```python
from build123d import *

# Parameters (mm, degrees)
SKETCH1_R           = 1.5
BOSS_EXTRUDE1_DEPTH = 3
SKETCH3_R           = 8.6
CUT_EXTRUDE2_DEPTH  = 4
SKETCH4_R           = 1.5
SKETCH4_R_2         = 1.475
CUT_EXTRUDE3_DEPTH  = 4
CUT_EXTRUDE4_DEPTH  = 4
CUT_EXTRUDE6_DEPTH  = 4
CUT_EXTRUDE7_DEPTH  = 4


with BuildPart() as part:
    # Sketch1 → Boss-Extrude1 (new body)
    with BuildSketch(Plane.XY):
        Polygon((0, -20.476245627), (7.465897773, -20.476245627), (9.02146997, -21.374355653), (9.387495374, -22.740381057), (11.136866689, -23.750381057), (15.4496732, -26.240381057), (21.596787517, -24.59326674), (32.096787517, -6.40673326), (30.4496732, -0.259618943), (26.136866689, 2.230381057), (24.387495374, 3.240381057), (23.02146997, 2.874355653), (21.465897773, 3.772465679), (17.732948887, 10.238122813), (14, 16.703779947), (14, 18.5), (15, 19.5), (15, 23), (15, 26.5), (10.5, 31), (-10.5, 31), (-15, 26.5), (-15, 23), (-15, 19.5), (-14, 18.5), (-14, 16.703779947), (-17.732948887, 10.238122813), (-21.465897773, 3.772465679), (-23.02146997, 2.874355653), (-24.387495374, 3.240381057), (-26.136866689, 2.230381057), (-30.4496732, -0.259618943), (-32.096787517, -6.40673326), (-21.596787517, -24.59326674), (-15.4496732, -26.240381057), (-11.136866689, -23.750381057), (-9.387495374, -22.740381057), (-9.02146997, -21.374355653), (-7.465897773, -20.476245627), align=None)
        with Locations((0, 23)):
            Circle(SKETCH1_R, mode=Mode.SUBTRACT)
        with Locations((19.918584287, -11.5)):
            Circle(SKETCH1_R, mode=Mode.SUBTRACT)
        with Locations((-19.918584287, -11.5)):
            Circle(SKETCH1_R, mode=Mode.SUBTRACT)
        Polygon((8, 23), (8, 25.75), (10, 25.75), (10, 23), (10, 20.25), (8, 20.25), align=None, mode=Mode.SUBTRACT)
        Polygon((12.537014427, -18.785254038), (13.636866689, -19.420254038), (17.300154147, -21.535254038), (18.300154147, -19.80320323), (15.918584287, -18.42820323), (13.537014427, -17.05320323), align=None, mode=Mode.SUBTRACT)
        Polygon((-8, 23), (-8, 20.25), (-10, 20.25), (-10, 23), (-10, 25.75), (-8, 25.75), align=None, mode=Mode.SUBTRACT)
        Polygon((27.300154147, -4.214745962), (23.636866689, -2.099745962), (22.537014427, -1.464745962), (21.537014427, -3.19679677), (23.918584287, -4.57179677), (26.300154147, -5.94679677), align=None, mode=Mode.SUBTRACT)
        Polygon((-22.537014427, -1.464745962), (-23.636866689, -2.099745962), (-27.300154147, -4.214745962), (-26.300154147, -5.94679677), (-23.918584287, -4.57179677), (-21.537014427, -3.19679677), align=None, mode=Mode.SUBTRACT)
        Polygon((-17.300154147, -21.535254038), (-13.636866689, -19.420254038), (-12.537014427, -18.785254038), (-13.537014427, -17.05320323), (-15.918584287, -18.42820323), (-18.300154147, -19.80320323), align=None, mode=Mode.SUBTRACT)
    extrude(amount=BOSS_EXTRUDE1_DEPTH)

    # Sketch3 → Cut-Extrude2 (cut, through all)
    with BuildSketch(Plane.XY.offset(3)):
        Circle(SKETCH3_R)
    extrude(amount=-CUT_EXTRUDE2_DEPTH, mode=Mode.SUBTRACT)

    # Sketch4 → Cut-Extrude3 (cut, through all)
    with BuildSketch(Plane.XY.offset(3)):
        with Locations((-7.5, -12.990381057)):
            Circle(SKETCH4_R)
        with Locations((-2.883414438, 11.648429988)):
            Circle(SKETCH4_R_2)
        with Locations((11.529543503, -3.327104841)):
            Circle(SKETCH4_R_2)
    extrude(amount=-CUT_EXTRUDE3_DEPTH, mode=Mode.SUBTRACT)

    # Sketch5 → Cut-Extrude4 (cut, through all)
    with BuildSketch(Plane.XY.offset(3)):
        with BuildLine():
            ThreePointArc((-5.590405789, -6.830501462), (-6.196392496, -5.963616355), (-7.039450485, -5.324896616))
            ThreePointArc((-7.039450485, -5.324896616), (-10.568748211, 3.049846104), (-3.120184892, 8.256684161))
            ThreePointArc((-3.120184892, 8.256684161), (-2.066447014, 8.348041491), (-1.0917705, 8.758791256))
            ThreePointArc((-1.0917705, 8.758791256), (7.925618309, 7.627881385), (8.710590681, -1.4261827))
            ThreePointArc((8.710590681, -1.4261827), (8.26283951, -2.384425136), (8.131220984, -3.433894641))
            ThreePointArc((8.131220984, -3.433894641), (2.643129902, -10.677727489), (-5.590405789, -6.830501462))
        make_face()
    extrude(amount=-CUT_EXTRUDE4_DEPTH, mode=Mode.SUBTRACT)

    # Sketch7 → Cut-Extrude6 (cut, through all)
    with BuildSketch(Plane.XY.offset(3)):
        with BuildLine():
            Line((12.279936491, 14.683017338), (18.855834264, 3.293228289))
            ThreePointArc((18.855834264, 3.293228289), (18.94474564, 2.617879339), (18.530071655, 2.077465679))
            Line((18.530071655, 2.077465679), (16.174482556, 0.717465679))
            ThreePointArc((16.174482556, 0.717465679), (15.499133606, 0.628554303), (14.958719947, 1.043228289))
            Line((14.958719947, 1.043228289), (8.382822174, 12.433017338))
            ThreePointArc((8.382822174, 12.433017338), (8.293910797, 13.108366288), (8.708584783, 13.648779947))
            Line((8.708584783, 13.648779947), (11.064173881, 15.008779947))
            ThreePointArc((11.064173881, 15.008779947), (11.739522831, 15.097691323), (12.279936491, 14.683017338))
        make_face()
        with BuildLine():
            Line((-12.279936491, 14.683017338), (-18.855834264, 3.293228289))
            ThreePointArc((-18.855834264, 3.293228289), (-18.94474564, 2.617879339), (-18.530071655, 2.077465679))
            Line((-18.530071655, 2.077465679), (-16.174482556, 0.717465679))
            ThreePointArc((-16.174482556, 0.717465679), (-15.499133606, 0.628554303), (-14.958719947, 1.043228289))
            Line((-14.958719947, 1.043228289), (-8.382822174, 12.433017338))
            ThreePointArc((-8.382822174, 12.433017338), (-8.293910797, 13.108366288), (-8.708584783, 13.648779947))
            Line((-8.708584783, 13.648779947), (-11.064173881, 15.008779947))
            ThreePointArc((-11.064173881, 15.008779947), (-11.739522831, 15.097691323), (-12.279936491, 14.683017338))
        make_face()
    extrude(amount=-CUT_EXTRUDE6_DEPTH, mode=Mode.SUBTRACT)

    # Sketch8 → Cut-Extrude7 (cut, through all)
    with BuildSketch(Plane.XY.offset(3)):
        Polygon((-3.538119785, -20.476245627), (-4, -19.676245627), (-4.461880215, -20.476245627), align=None)
    extrude(amount=-CUT_EXTRUDE7_DEPTH, mode=Mode.SUBTRACT)


solid = part.part
```
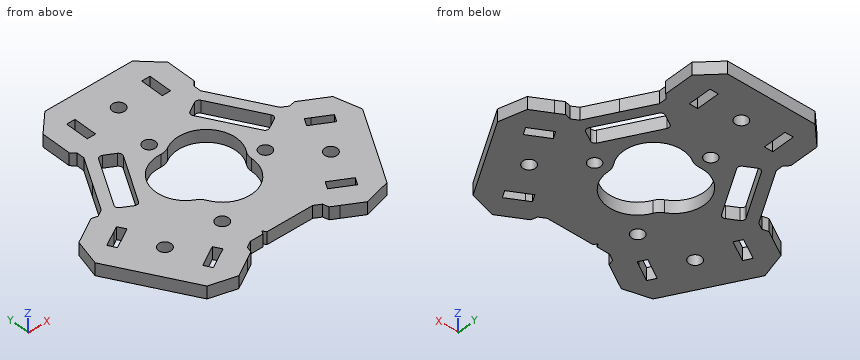
Can you work these out from the model? Positions are in its coordinate system, mm. Coordinates: 2 decimals unless noted, no trailing zeros. Order: outer loops, then holes, each group sorted by start corner. A loop starts at its lowest first (then second) coordinate and runs counter-clockwise, first axis right, second up.
1. If we section it at A-A (y = 23): Please give me the cut outline in (x, z), then the cut area to 3 significant figures.
2. If we section it at B-B (x = 5.5): Please give me the cut outline in (y, z).
3. I need wall thicknesses on line 1 (X direction, y = 14, z = 0.7); line 2 (Y direction, x = 0, z = 1.65); line 3 (X direction, y = 9, z = 1.55). Which ranges of each line are inside material? Lowest first, please.
4. I'm going to push flat-ended pins straight in: pin 1 (1 mm diameter, centred on y = 11.5, z = 0.5, fed in from +X); pin 2 (1.5 mm diameter, centred on y = 23.5, z = 1, fed in from +X); pin 3 (1.5 mm diameter, centred on y = 16.5, z = 1.5, fed in from +X); pin 4 (2.5 mm diameter, centred on x = -19.92, y = -11.5, fed in from -Z). Where does each tip first touch, or does it pass through?
5. If we section it at C-C (z = 2.5): Give the number of separate pieces and of enclosed holes in the cut face, then the cut area to 3 significant figures.
Entries:
1. outline: (-15, 0) - (-10, 0) - (-10, 3) - (-15, 3) - close; (-8, 0) - (-1.5, 0) - (-1.5, 3) - (-8, 3) - close; (1.5, 0) - (8, 0) - (8, 3) - (1.5, 3) - close; (10, 0) - (15, 0) - (15, 3) - (10, 3) - close
1. area: 69.0 mm2
2. outline: (-20.48, 0) - (-9.24, 0) - (-9.24, 3) - (-20.48, 3) - close; (9.29, 0) - (31, 0) - (31, 3) - (9.29, 3) - close
3. line 1: x = -15.56 to -12.67, -9.32 to 9.32, 12.67 to 15.56
3. line 2: y = -20.48 to -10.83, 9.31 to 21.5, 24.5 to 31
3. line 3: x = -18.45 to -15.56, -10.36 to -0.67, 6.11 to 10.36, 15.56 to 18.45
4. pin 1: stops at x = 17.29
4. pin 2: stops at x = 15
4. pin 3: stops at x = 14.55
4. pin 4: passes through
5. separate pieces: 1
5. enclosed holes: 15
5. area: 1,810 mm2
